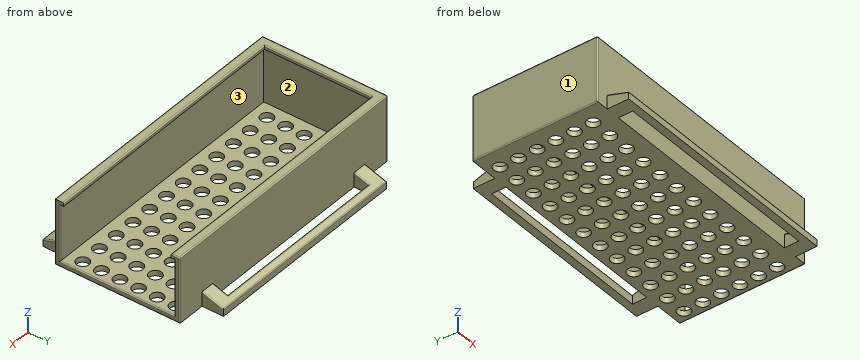
```python
from build123d import *

# Parameters (mm, degrees)
SKETCH_1_W          = 74.5
SKETCH_1_H          = 34.9
SKETCH_1_W_2        = 71.5
SKETCH_1_H_2        = 31.9
EXTRUDE_1_DEPTH     = 18.2
SKETCH_2_W          = 71.5
SKETCH_2_H          = 31.9
EXTRUDE_2_DEPTH     = 1.5
SKETCH_3_W          = 16.7
SKETCH_3_H          = 31.9
CUT_EXTRUDE_1_DEPTH = 83.315247676
EXTRUDE_3_DEPTH     = 1
SKETCH_5_W          = 4
SKETCH_5_H          = 4
EXTRUDE_5_DEPTH     = 6
EXTRUDE_6_REACH     = 78.091
SKETCH_15_W         = 4
SKETCH_15_H         = 2
CUT_EXTRUDE_2_DEPTH = 80.409382317
SKETCH_17_W         = 4
SKETCH_17_H         = 4
EXTRUDE_7_DEPTH     = 6
EXTRUDE_8_REACH     = 81.829
SKETCH_18_W         = 4
SKETCH_18_H         = 2
CUT_EXTRUDE_3_DEPTH = 84.214181484
FILLET_1_R          = 0.3
SKETCH_20_R         = 1.75
CUT_EXTRUDE_4_DEPTH = 85.618260441


with BuildPart() as part:
    # 草图1 → 凸台-拉伸1 (new body)
    with BuildSketch(Plane.XY):
        with Locations((35.75, 15.95)):
            Rectangle(SKETCH_1_W, SKETCH_1_H)
        with Locations((35.75, 15.95)):
            Rectangle(SKETCH_1_W_2, SKETCH_1_H_2, mode=Mode.SUBTRACT)
    extrude(amount=EXTRUDE_1_DEPTH)

    # 草图2 → 凸台-拉伸2 (add)
    with BuildSketch(Plane(origin=(0, 0, 0), x_dir=(-1, 0, 0), z_dir=(0, 0, -1))):
        with Locations((-35.75, 15.95)):
            Rectangle(SKETCH_2_W, SKETCH_2_H)
    extrude(amount=-EXTRUDE_2_DEPTH)

    # 草图3 → 切除-拉伸1 (cut, through all)
    with BuildSketch(Plane.ZY.offset(-71.5)):
        with Locations((9.85, 15.95)):
            Rectangle(SKETCH_3_W, SKETCH_3_H)
    extrude(amount=-CUT_EXTRUDE_1_DEPTH, mode=Mode.SUBTRACT)

    # 草图4 → 凸台-拉伸3 (add)
    with BuildSketch(Plane.XY.offset(18.2)):
        Polygon((1, 1), (73, 1), (73, 0), (0, 0), (0, 31.9), (73, 31.9), (73, 30.9), (1, 30.9), align=None)
    extrude(amount=-EXTRUDE_3_DEPTH)

    # 草图5 → 凸台-拉伸5 (add)
    with BuildSketch(Plane(origin=(0, 33.4, 0), x_dir=(1, 0, 0), z_dir=(0, 1, 0))):
        with Locations((8.5, -2)):
            Rectangle(SKETCH_5_W, SKETCH_5_H)
        with Locations((63, -2)):
            Rectangle(SKETCH_5_W, SKETCH_5_H)
    extrude(amount=EXTRUDE_5_DEPTH)

    # 草图15 → 凸台-拉伸6 (add, up to next)
    with BuildSketch(Plane.ZY.offset(-61), mode=Mode.PRIVATE) as extrude_6_sk1:
        with Locations((2, 38.4)):
            Rectangle(SKETCH_15_W, SKETCH_15_H)
    extrude_6_tool1 = extrude(extrude_6_sk1.sketch, amount=EXTRUDE_6_REACH, mode=Mode.PRIVATE) - part.part
    add(extrude_6_tool1.solids().sort_by_distance((61, 38.4, 2))[0])

    # 草图16 → 切除-拉伸2 (cut, through all)
    with BuildSketch(Plane(origin=(65, 0, 0), x_dir=(0, 0, -1), z_dir=(1, 0, 0))):
        Polygon((-4, 33.4), (-2, 39.4), (-4, 39.4), align=None)
    extrude(amount=-CUT_EXTRUDE_2_DEPTH, mode=Mode.SUBTRACT)

    # 草图17 → 凸台-拉伸7 (add)
    with BuildSketch(Plane.XZ.offset(1.5)):
        with Locations((4, 2)):
            Rectangle(SKETCH_17_W, SKETCH_17_H)
        with Locations((67.5, 2)):
            Rectangle(SKETCH_17_W, SKETCH_17_H)
    extrude(amount=EXTRUDE_7_DEPTH)

    # 草图18 → 凸台-拉伸8 (add, up to next)
    with BuildSketch(Plane.ZY.offset(-65.5), mode=Mode.PRIVATE) as extrude_8_sk1:
        with Locations((2, -6.5)):
            Rectangle(SKETCH_18_W, SKETCH_18_H)
    extrude_8_tool1 = extrude(extrude_8_sk1.sketch, amount=EXTRUDE_8_REACH, mode=Mode.PRIVATE) - part.part
    add(extrude_8_tool1.solids().sort_by_distance((65.5, -6.5, 2))[0])

    # 草图19 → 切除-拉伸3 (cut, through all)
    with BuildSketch(Plane.ZY.offset(-2)):
        Polygon((4, -1.5), (2, -7.5), (4, -7.5), align=None)
    extrude(amount=-CUT_EXTRUDE_3_DEPTH, mode=Mode.SUBTRACT)

    # 圆角1
    fillet_1_edges = [part.edges().sort_by_distance(p)[0] for p in [
        (-1.5, 33.4, 9.1),
        (-1.5, 15.95, 18.2),
        (-1.5, -1.5, 9.1),
        (-1.5, 15.95, 0),
        (73, 31.9, 9.35),
        (73, 15.95, 1.5),
        (73, 0, 9.35),
        (73, -1.5, 9.1),
        (1, 15.95, 18.2),
        (37, 1, 18.2),
        (35.75, -1.5, 18.2),
        (73, 15.95, 0),
        (73, 32.15, 18.2),
        (37, 30.9, 18.2),
        (73, 33.4, 9.1),
        (35.75, 33.4, 18.2),
        (10.5, 35.4, 3.333333333),
        (35.75, 37.4, 2.666666667),
        (61, 35.4, 3.333333333),
        (6, -3.5, 3.333333333),
        (35.75, -5.5, 2.666666667),
        (65.5, -3.5, 3.333333333),
        (69.5, -4.5, 3),
        (35.75, -7.5, 2),
        (2, -4.5, 3),
        (65, 36.4, 3),
        (35.75, 39.4, 2),
        (6.5, 36.4, 3),
    ]]
    fillet(fillet_1_edges, radius=FILLET_1_R)

    # 草图20 → 切除-拉伸4 (cut, through all)
    with BuildSketch(Plane.XY.offset(1.5)):
        with Locations((4, 4)):
            Circle(SKETCH_20_R)
        with Locations((10, 4)):
            Circle(SKETCH_20_R)
        with Locations((16, 4)):
            Circle(SKETCH_20_R)
        with Locations((22, 4)):
            Circle(SKETCH_20_R)
        with Locations((28, 4)):
            Circle(SKETCH_20_R)
        with Locations((34, 4)):
            Circle(SKETCH_20_R)
        with Locations((40, 4)):
            Circle(SKETCH_20_R)
        with Locations((46, 4)):
            Circle(SKETCH_20_R)
        with Locations((52, 4)):
            Circle(SKETCH_20_R)
        with Locations((58, 4)):
            Circle(SKETCH_20_R)
        with Locations((64, 4)):
            Circle(SKETCH_20_R)
        with Locations((70, 4)):
            Circle(SKETCH_20_R)
        with Locations((4, 9.2)):
            Circle(SKETCH_20_R)
        with Locations((4, 14.4)):
            Circle(SKETCH_20_R)
        with Locations((4, 19.6)):
            Circle(SKETCH_20_R)
        with Locations((4, 24.8)):
            Circle(SKETCH_20_R)
        with Locations((4, 30)):
            Circle(SKETCH_20_R)
        with Locations((10, 30)):
            Circle(SKETCH_20_R)
        with Locations((10, 24.8)):
            Circle(SKETCH_20_R)
        with Locations((10, 19.6)):
            Circle(SKETCH_20_R)
        with Locations((10, 14.4)):
            Circle(SKETCH_20_R)
        with Locations((10, 9.2)):
            Circle(SKETCH_20_R)
        with Locations((16, 30)):
            Circle(SKETCH_20_R)
        with Locations((16, 24.8)):
            Circle(SKETCH_20_R)
        with Locations((16, 19.6)):
            Circle(SKETCH_20_R)
        with Locations((16, 14.4)):
            Circle(SKETCH_20_R)
        with Locations((16, 9.2)):
            Circle(SKETCH_20_R)
        with Locations((22, 30)):
            Circle(SKETCH_20_R)
        with Locations((22, 24.8)):
            Circle(SKETCH_20_R)
        with Locations((22, 19.6)):
            Circle(SKETCH_20_R)
        with Locations((22, 14.4)):
            Circle(SKETCH_20_R)
        with Locations((22, 9.2)):
            Circle(SKETCH_20_R)
        with Locations((28, 30)):
            Circle(SKETCH_20_R)
        with Locations((28, 24.8)):
            Circle(SKETCH_20_R)
        with Locations((28, 19.6)):
            Circle(SKETCH_20_R)
        with Locations((28, 14.4)):
            Circle(SKETCH_20_R)
        with Locations((28, 9.2)):
            Circle(SKETCH_20_R)
        with Locations((34, 30)):
            Circle(SKETCH_20_R)
        with Locations((34, 24.8)):
            Circle(SKETCH_20_R)
        with Locations((34, 19.6)):
            Circle(SKETCH_20_R)
        with Locations((34, 14.4)):
            Circle(SKETCH_20_R)
        with Locations((34, 9.2)):
            Circle(SKETCH_20_R)
        with Locations((40, 30)):
            Circle(SKETCH_20_R)
        with Locations((40, 24.8)):
            Circle(SKETCH_20_R)
        with Locations((40, 19.6)):
            Circle(SKETCH_20_R)
        with Locations((40, 14.4)):
            Circle(SKETCH_20_R)
        with Locations((40, 9.2)):
            Circle(SKETCH_20_R)
        with Locations((46, 30)):
            Circle(SKETCH_20_R)
        with Locations((46, 24.8)):
            Circle(SKETCH_20_R)
        with Locations((46, 19.6)):
            Circle(SKETCH_20_R)
        with Locations((46, 14.4)):
            Circle(SKETCH_20_R)
        with Locations((46, 9.2)):
            Circle(SKETCH_20_R)
        with Locations((52, 30)):
            Circle(SKETCH_20_R)
        with Locations((52, 24.8)):
            Circle(SKETCH_20_R)
        with Locations((52, 19.6)):
            Circle(SKETCH_20_R)
        with Locations((52, 14.4)):
            Circle(SKETCH_20_R)
        with Locations((52, 9.2)):
            Circle(SKETCH_20_R)
        with Locations((58, 30)):
            Circle(SKETCH_20_R)
        with Locations((58, 24.8)):
            Circle(SKETCH_20_R)
        with Locations((58, 19.6)):
            Circle(SKETCH_20_R)
        with Locations((58, 14.4)):
            Circle(SKETCH_20_R)
        with Locations((58, 9.2)):
            Circle(SKETCH_20_R)
        with Locations((64, 30)):
            Circle(SKETCH_20_R)
        with Locations((64, 24.8)):
            Circle(SKETCH_20_R)
        with Locations((64, 19.6)):
            Circle(SKETCH_20_R)
        with Locations((64, 14.4)):
            Circle(SKETCH_20_R)
        with Locations((64, 9.2)):
            Circle(SKETCH_20_R)
        with Locations((70, 30)):
            Circle(SKETCH_20_R)
        with Locations((70, 24.8)):
            Circle(SKETCH_20_R)
        with Locations((70, 19.6)):
            Circle(SKETCH_20_R)
        with Locations((70, 14.4)):
            Circle(SKETCH_20_R)
        with Locations((70, 9.2)):
            Circle(SKETCH_20_R)
    extrude(amount=-CUT_EXTRUDE_4_DEPTH, mode=Mode.SUBTRACT)


solid = part.part
```
The model under review builds one solid part; all positions refer to its coordinate system, in mm. Face numbers are marked on the shaded views. Coordinates: 2 decimals unless noted, no trailing zeros. Write each loop counter-clockwise with the first axis right and the second up, starting at its lowest first coordinate (ties: lowest second). Pieces come first, ordered by that corner, then holes. Notation, with made-up numbers: (41.5, 46.5) -> (61.5, 46.5) arc R32 cw to (61.5, 84.5) -> close; hole circle Ø4 at (68.5, 45). An arc over 180 degrees is marked (long way). One line per item, written item: value. Start each with the question number.
Q1. Clearance check with flat-ended pins moving along their axes: P1, Ø4, axis at x = 34, y = 4, coming from the +Z side; P2, Ø5.5, axis at x = 51, z = 10, coming from the -Y side. State where each tip first meets the part, or that it passes through.
Q2. Add section B-B, the plane y = 4. Count the separate pieces of the cut face and the enclosed holes in it, then the cut area to 3 significant figures.
Q3. The part is to be moulded in two halves that separate along Y. For the marked faces 1, 2 and 3, say which applies: +Y half, -Y half, draft (parallel to the pull), parting line (faces both ways), or undercut.
Q4. To check wall thickness, follow probe 1 along Y at (x, z) = (48, 17.75); probe 2 along Y at (x, z) = (39, 5.25); probe 3 along Z at (x, y) = (57.5, 0.5). State the ranges of each line that lie inside material, in increasing order.
Q5. Add section A-A, the plane z = 16. Give the boundary of the cut face in (x, y), then the cut area to 3 significant figures.
Response:
1. P1: z = 1.5
1. P2: y = -1.5
2. separate pieces: 13
2. enclosed holes: 0
2. area: 74.7 mm²
3. face 1: draft
3. face 2: undercut
3. face 3: undercut
4. probe 1: -1.5 to 1, 30.9 to 33.4
4. probe 2: -1.5 to 0, 31.9 to 33.4
4. probe 3: 0 to 1.5, 17.2 to 18.2
5. outline: (-1.5, -1.2) arc R0.3 ccw to (-1.2, -1.5) -> (72.7, -1.5) arc R0.3 ccw to (73, -1.2) -> (73, -0.3) arc R0.3 ccw to (72.7, 0) -> (0, 0) -> (0, 31.9) -> (72.7, 31.9) arc R0.3 ccw to (73, 32.2) -> (73, 33.1) arc R0.3 ccw to (72.7, 33.4) -> (-1.2, 33.4) arc R0.3 ccw to (-1.5, 33.1) -> close
5. area: 271 mm²
